Can you work these out from the model? Positions are in its coordinate system, mm. A direction names the side the tool comes from. Round coordinates to 2 decimals unless told otherwise and drop trailing zeros. Write each loop counter-clockwise with the first axis right and the second up, starting at its lowest first coordinate (ties: lowest second). Pieces come first, ordered by that corner, then holes. Notation, with made-up numbers: M -10,36.5 L 35,36.5 A17 cw 35,49.5 Z; hole C 12,61.5 d8. An arc over 180 degrees is marked long. Answer as a JSON object with one key per item and string values. Group by question number.
1) Suppose I cut it at D-D, the plane z = 30.5. Write out the boundary of the cut face in (x, y), and give its area (3 significant figures).
2) On a 3-axis mill with a long thin cutter (end or side, diameter ignored), from which of +Z, -Z, +X, -X, +Y, -Y can I reach the whole of each face in a straight line? I mean faces 4 (the cylindrical face through (5.672, 5.641, 8.656)), 5 (the cylindrical face through (2.098, -2.145, 0.986)), 6 (the cylindrical face through (-0.596, -2.685, 28.958)). Say none if no direction works.
3) Suppose I cut it at B-B, the plane x = 0. Write out the boundary of the cut face in (y, z), and give its area (3 significant figures).
4) Suppose I cut it at A-A, the plane z = 12.5. Write out the boundary of the cut face in (x, y).
5) I'm going to push flat-ended pins straight in: pin 1 Ø2.5 at (x, y) = (-4.5, -3.5) entering from -Z; pin 2 Ø7 at (y, z) = (-2, 8) entering from +X; pin 3 Ø8 at (x, z) = (-1, 6) entering from +Y; pin 4 Ø1.6 at (y, z) = (0, 12.5) entering from -X. Where does each tip first touch, or does it pass through?
6) If we mould it in two halves opening along Y, with no side actions, what happens to faces 1 (the cylindrical face through (-5.672, -5.641, 8.656)), 2 (the flat face through (0, 0, 17)), 3 (the flat face through (4, 4, 2))? For each: +Y half, -Y half, draft (parallel to the pull), parting line (faces both ways), or undercut.
7) Suppose I cut it at C-C, the plane y = -0.5. Write out the boundary of the cut face in (x, z), and give its area (3 significant figures).
8) Please list where these lines run through material, in increasing order: L1, parallel to Z at x = -3, y = 0; L2, parallel to Y at x = 0, z = 27.25; L3, parallel to Z at x = 2, y = 0. Write a range as [from, to].
from build123d import *

# Parameters (mm, degrees)
BOSS_EXTRUDE3_START = 5.5
SKETCH3_R           = 9
BOSS_EXTRUDE3_DEPTH = 3
SKETCH4_R           = 5.75
BOSS_EXTRUDE4_DEPTH = 7.5
SKETCH5_R           = 2.75
BOSS_EXTRUDE5_DEPTH = 6
BOSS_EXTRUDE8_DEPTH = 2
BOSS_EXTRUDE9_START = 2
SKETCH1_7_R         = 2
BOSS_EXTRUDE9_DEPTH = 13.5
SKETCH6_R           = 1
CUT_EXTRUDE1_DEPTH  = 15
CHAMFER1_SIZE       = 0.5
SKETCH7_R           = 1.75
CUT_EXTRUDE2_DEPTH  = 15


with BuildPart() as part:
    # Sketch3 → Boss-Extrude3 (new body)
    with BuildSketch(Plane.XY.offset(10).offset(BOSS_EXTRUDE3_START)):
        Circle(SKETCH3_R)
    extrude(amount=BOSS_EXTRUDE3_DEPTH)

    # Sketch4 → Boss-Extrude4 (add)
    with BuildSketch(Plane.XY.offset(18.5)):
        with Locations((0, -1.812)):
            Circle(SKETCH4_R)
    extrude(amount=BOSS_EXTRUDE4_DEPTH)

    # Sketch5 → Boss-Extrude5 (add)
    with BuildSketch(Plane.XY.offset(26)):
        Circle(SKETCH5_R)
    extrude(amount=BOSS_EXTRUDE5_DEPTH)



with BuildPart() as body_2:
    # Sketch1 → Boss-Extrude8 (new body)
    with BuildSketch(Plane.XY):
        with BuildLine():
            Line((1.242640687, 4.242640687), (1.242640687, 6.242640687))
            Line((1.242640687, 6.242640687), (-1.242640687, 6.242640687))
            Line((-1.242640687, 6.242640687), (-1.242640687, 4.242640687))
            ThreePointArc((-1.242640687, 4.242640687), (-2.121320344, 2.121320343), (-4.242640687, 1.242640687))
            Line((-4.242640687, 1.242640687), (-6.242640687, 1.242640687))
            Line((-6.242640687, 1.242640687), (-6.242640687, -1.242640687))
            Line((-6.242640687, -1.242640687), (-4.242640687, -1.242640687))
            ThreePointArc((-4.242640687, -1.242640687), (-2.121320343, -2.121320344), (-1.242640687, -4.242640687))
            Line((-1.242640687, -4.242640687), (-1.242640687, -6.242640687))
            Line((-1.242640687, -6.242640687), (1.242640687, -6.242640687))
            Line((1.242640687, -6.242640687), (1.242640687, -4.242640687))
            ThreePointArc((1.242640687, -4.242640687), (2.121320344, -2.121320343), (4.242640687, -1.242640687))
            Line((4.242640687, -1.242640687), (6.242640687, -1.242640687))
            Line((6.242640687, -1.242640687), (6.242640687, 1.242640687))
            Line((6.242640687, 1.242640687), (4.242640687, 1.242640687))
            ThreePointArc((4.242640687, 1.242640687), (2.121320343, 2.121320344), (1.242640687, 4.242640687))
        make_face()
    extrude(amount=BOSS_EXTRUDE8_DEPTH)


with BuildPart() as part_1:
    add(part.part)

    add(body_2.part)  # Boss-Extrude9 merges body 2
    # Sketch1_7 → Boss-Extrude9 (add)
    with BuildSketch(Plane.XY.offset(BOSS_EXTRUDE9_START)):
        with BuildLine():
            Line((1.242640687, 4.242640687), (1.242640687, 6.242640687))
            Line((1.242640687, 6.242640687), (-1.242640687, 6.242640687))
            Line((-1.242640687, 6.242640687), (-1.242640687, 4.242640687))
            ThreePointArc((-1.242640687, 4.242640687), (-2.121320344, 2.121320343), (-4.242640687, 1.242640687))
            Line((-4.242640687, 1.242640687), (-6.242640687, 1.242640687))
            Line((-6.242640687, 1.242640687), (-6.242640687, -1.242640687))
            Line((-6.242640687, -1.242640687), (-4.242640687, -1.242640687))
            ThreePointArc((-4.242640687, -1.242640687), (-2.121320343, -2.121320344), (-1.242640687, -4.242640687))
            Line((-1.242640687, -4.242640687), (-1.242640687, -6.242640687))
            Line((-1.242640687, -6.242640687), (1.242640687, -6.242640687))
            Line((1.242640687, -6.242640687), (1.242640687, -4.242640687))
            ThreePointArc((1.242640687, -4.242640687), (2.121320344, -2.121320343), (4.242640687, -1.242640687))
            Line((4.242640687, -1.242640687), (6.242640687, -1.242640687))
            Line((6.242640687, -1.242640687), (6.242640687, 1.242640687))
            Line((6.242640687, 1.242640687), (4.242640687, 1.242640687))
            ThreePointArc((4.242640687, 1.242640687), (2.121320343, 2.121320344), (1.242640687, 4.242640687))
        make_face()
        with BuildLine():
            Line((-1.242640687, 4.242640687), (-1.242640687, 6.242640687))
            Line((-1.242640687, 6.242640687), (-2.242640687, 6.242640687))
            Line((-2.242640687, 6.242640687), (-2.242640687, 4.242640687))
            ThreePointArc((-2.242640687, 4.242640687), (-2.828427125, 2.828427125), (-4.242640687, 2.242640687))
            Line((-4.242640687, 2.242640687), (-6.242640687, 2.242640687))
            Line((-6.242640687, 2.242640687), (-6.242640687, 1.242640687))
            Line((-6.242640687, 1.242640687), (-4.242640687, 1.242640687))
            ThreePointArc((-4.242640687, 1.242640687), (-2.121320344, 2.121320343), (-1.242640687, 4.242640687))
        make_face()
        with BuildLine():
            Line((2.242640687, 4.242640687), (2.242640687, 6.242640687))
            Line((2.242640687, 6.242640687), (1.242640687, 6.242640687))
            Line((1.242640687, 6.242640687), (1.242640687, 4.242640687))
            ThreePointArc((1.242640687, 4.242640687), (2.121320343, 2.121320344), (4.242640687, 1.242640687))
            Line((4.242640687, 1.242640687), (6.242640687, 1.242640687))
            Line((6.242640687, 1.242640687), (6.242640687, 2.242640687))
            Line((6.242640687, 2.242640687), (4.242640687, 2.242640687))
            ThreePointArc((4.242640687, 2.242640687), (2.828427124, 2.828427125), (2.242640687, 4.242640687))
        make_face()
        with BuildLine():
            Line((6.242640687, -2.242640687), (6.242640687, -1.242640687))
            Line((6.242640687, -1.242640687), (4.242640687, -1.242640687))
            ThreePointArc((4.242640687, -1.242640687), (2.121320344, -2.121320343), (1.242640687, -4.242640687))
            Line((1.242640687, -4.242640687), (1.242640687, -6.242640687))
            Line((1.242640687, -6.242640687), (2.242640687, -6.242640687))
            Line((2.242640687, -6.242640687), (2.242640687, -4.242640687))
            ThreePointArc((2.242640687, -4.242640687), (2.828427125, -2.828427125), (4.242640687, -2.242640687))
            Line((4.242640687, -2.242640687), (6.242640687, -2.242640687))
        make_face()
        with BuildLine():
            Line((-4.242640687, -1.242640687), (-6.242640687, -1.242640687))
            Line((-6.242640687, -1.242640687), (-6.242640687, -2.242640687))
            Line((-6.242640687, -2.242640687), (-4.242640687, -2.242640687))
            ThreePointArc((-4.242640687, -2.242640687), (-2.828427125, -2.828427125), (-2.242640687, -4.242640687))
            Line((-2.242640687, -4.242640687), (-2.242640687, -6.242640687))
            Line((-2.242640687, -6.242640687), (-1.242640687, -6.242640687))
            Line((-1.242640687, -6.242640687), (-1.242640687, -4.242640687))
            ThreePointArc((-1.242640687, -4.242640687), (-2.121320343, -2.121320344), (-4.242640687, -1.242640687))
        make_face()
        with BuildLine():
            Line((-4.242640687, -2.242640687), (-6.242640687, -2.242640687))
            Line((-6.242640687, -2.242640687), (-6.242640687, -4.242640687))
            ThreePointArc((-6.242640687, -4.242640687), (-5.656854249, -2.828427125), (-4.242640687, -2.242640687))
        make_face()
        with Locations((-4.242640687, -4.242640687)):
            Circle(SKETCH1_7_R)
        with BuildLine():
            Line((-4.242640687, -6.242640687), (-2.242640687, -6.242640687))
            Line((-2.242640687, -6.242640687), (-2.242640687, -4.242640687))
            ThreePointArc((-2.242640687, -4.242640687), (-2.828427125, -5.656854249), (-4.242640687, -6.242640686))
        make_face()
        with BuildLine():
            Line((2.242640687, -6.242640687), (4.242640687, -6.242640687))
            ThreePointArc((4.242640687, -6.242640686), (2.828427125, -5.656854249), (2.242640687, -4.242640687))
            Line((2.242640687, -4.242640687), (2.242640687, -6.242640687))
        make_face()
        with Locations((4.242640687, -4.242640687)):
            Circle(SKETCH1_7_R)
        with BuildLine():
            Line((6.242640687, -4.242640687), (6.242640687, -2.242640687))
            Line((6.242640687, -2.242640687), (4.242640687, -2.242640687))
            ThreePointArc((4.242640687, -2.242640687), (5.656854249, -2.828427125), (6.242640686, -4.242640687))
        make_face()
        with Locations((4.242640687, 4.242640687)):
            Circle(SKETCH1_7_R)
        with BuildLine():
            Line((6.242640687, 2.242640687), (6.242640687, 4.242640687))
            ThreePointArc((6.242640687, 4.242640687), (5.656854249, 2.828427125), (4.242640687, 2.242640687))
            Line((4.242640687, 2.242640687), (6.242640687, 2.242640687))
        make_face()
        with BuildLine():
            ThreePointArc((2.242640687, 4.242640687), (2.828427124, 5.656854249), (4.242640687, 6.242640687))
            Line((4.242640687, 6.242640687), (2.242640687, 6.242640687))
            Line((2.242640687, 6.242640687), (2.242640687, 4.242640687))
        make_face()
        with BuildLine():
            Line((-2.242640687, 4.242640687), (-2.242640687, 6.242640687))
            Line((-2.242640687, 6.242640687), (-4.242640687, 6.242640687))
            ThreePointArc((-4.242640687, 6.242640687), (-2.828427125, 5.656854249), (-2.242640687, 4.242640687))
        make_face()
        with Locations((-4.242640687, 4.242640687)):
            Circle(SKETCH1_7_R)
        with BuildLine():
            ThreePointArc((-4.242640687, 2.242640687), (-5.656854249, 2.828427125), (-6.242640687, 4.242640687))
            Line((-6.242640687, 4.242640687), (-6.242640687, 2.242640687))
            Line((-6.242640687, 2.242640687), (-4.242640687, 2.242640687))
        make_face()
    extrude(amount=BOSS_EXTRUDE9_DEPTH)

    # Sketch6 → Cut-Extrude1 (cut)
    with BuildSketch(Plane(origin=(6.242640687, 0, 0), x_dir=(0, 0, -1), z_dir=(1, 0, 0))):
        with Locations(Location((-12.5, 0, 0), (0, 0, 90))):
            Circle(SKETCH6_R)
    extrude(amount=-CUT_EXTRUDE1_DEPTH, mode=Mode.SUBTRACT)

    # Chamfer1
    chamfer1_edges = [part_1.edges().sort_by_distance(p)[0] for p in [
        (-6.242640687, 0, 0),
        (0, 6.242640687, 0),
        (6.242640687, 0, 0),
        (0, -6.242640687, 0),
    ]]
    chamfer(chamfer1_edges, length=CHAMFER1_SIZE)

    # Sketch7 → Cut-Extrude2 (cut)
    with BuildSketch(Plane.XY.offset(32)):
        Circle(SKETCH7_R)
    extrude(amount=-CUT_EXTRUDE2_DEPTH, mode=Mode.SUBTRACT)


solid = part_1.part
Results:
{
 "1": {"outline": "C 0,0 d5.5; hole C 0,0 d3.5", "area": "14.1 mm^2"},
 "2": {"face 4": "-Z, +X, +Y", "face 5": "-Z, +X, -Y", "face 6": "+Z"},
 "3": {"outline": "M -9,15.5 L -6.24,15.5 L -6.24,0.5 L -5.74,0 L 5.74,0 L 6.24,0.5 L 6.24,15.5 L 9,15.5 L 9,18.5 L 3.94,18.5 L 3.94,26 L 2.75,26 L 2.75,32 L 1.75,32 L 1.75,17 L -1.75,17 L -1.75,32 L -2.75,32 L -2.75,26 L -7.56,26 L -7.56,18.5 L -9,18.5 Z; hole C 0,12.5 d2", "area": "311 mm^2"},
 "4": {"outline": "M -6.24,-4.24 A2 ccw -4.24,-6.24 L 4.24,-6.24 A2 ccw 6.24,-4.24 L 6.24,-1 L -6.24,-1 Z; M -6.24,1 L 6.24,1 L 6.24,4.24 A2 ccw 4.24,6.24 L -4.24,6.24 A2 ccw -6.24,4.24 Z"},
 "5": {"pin 1": "z = 2", "pin 2": "x = 6.24", "pin 3": "y = 6.24", "pin 4": "through"},
 "6": {"face 1": "-Y half", "face 2": "undercut", "face 3": "draft"},
 "7": {"outline": "M -8.99,15.5 L -6.24,15.5 L -6.24,13.37 L 6.24,13.37 L 6.24,15.5 L 8.99,15.5 L 8.99,18.5 L 5.6,18.5 L 5.6,26 L 2.7,26 L 2.7,32 L 1.68,32 L 1.68,17 L -1.68,17 L -1.68,32 L -2.7,32 L -2.7,26 L -5.6,26 L -5.6,18.5 L -8.99,18.5 Z; M -6.24,0.5 L -5.74,0 L 5.74,0 L 6.24,0.5 L 6.24,11.63 L -6.24,11.63 Z", "area": "292 mm^2"},
 "8": {"L1": "[0, 11.5], [13.5, 26]", "L2": "[-2.75, -1.75], [1.75, 2.75]", "L3": "[0, 11.5], [13.5, 32]"}
}
